For this review, take the finished solid that the model builds, in its own axes (mm). Give positions to 0.01 mm unless a question says otherwise; leave off trailing zeros. Order: outer loops, then holes, each group sorted by start corner. A loop starts at its lowest first (then second) coordinate and runs counter-clockwise, first axis right, second up.
Item 1: For probe 1 along Z at (x, y) = (1, 88.9); probe 2 along Z at (x, y) = (1.9, 17.5); probe 3 along Y at (x, z) = (3.65, -217.5), list the stretches that pass through material, from the lowest coordinate up.
Item 2: Consider section B-B (y = 88.9). Give the boundary of the cut face in (x, z).
Item 3: Consider section A-A (x = 1.8). Give the number of separate pieces and of enclosed holes in the cut face, plus the area to 3 significant figures.
Item 4: Consider section D-D (y = 50.5). Give the boundary of the cut face in (x, z).
Item 5: For P1, Ø1.5, axis at x = 1, z = -73.5, coming from the -Y side; P2, Ø1.2, axis at x = 2.5, y = -133.5, coming from the -Z side; P3, Ø2, axis at x = 1.5, z = -117, coming from the -Y side, all flat-tipped, find the tip position at first contact; note any pin that passes through.
Item 6: Consider section C-C (z = -44.45). Give the boundary of the cut face in (x, y), plus the area to 3 significant figures.
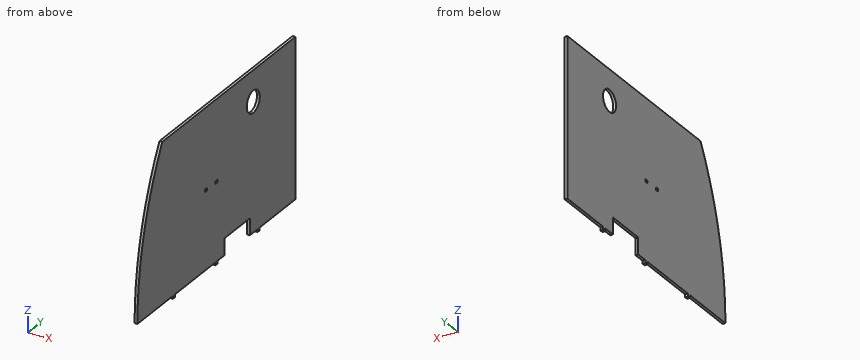
```python
from build123d import *

# Parameters (mm, degrees)
F0_R     = 15.6845
F1_DEPTH = 4.0894
F2_W     = 5.08
F2_H     = 4.0894
F3_DEPTH = 25.4


with BuildPart() as f1:
    # F0 (on Right) → F1 (new body)
    with BuildSketch(Plane.YZ):
        with BuildLine():
            Line((104.3824, -228.6), (190.5, -228.6))
            Line((190.5, -228.6), (190.5, 0))
            Line((190.5, 0), (-130.401722, 0))
            ThreePointArc((-130.401722, 0), (-175.224427, -110.416072), (-190.5, -228.6))
            Line((-190.5, -228.6), (-104.821593, -228.6))
            Line((-104.821593, -228.6), (-99.995593, -228.6))
            Line((-99.995593, -228.6), (-2.54, -228.6))
            Line((-2.54, -228.6), (-2.413, -228.6))
            Line((-2.413, -228.6), (2.413, -228.6))
            Line((2.413, -228.6), (2.54, -228.6))
            Line((2.54, -228.6), (19.796586, -228.6))
            Line((19.796586, -228.6), (19.796586, -204.705998))
            Line((19.796586, -204.705998), (80.546886, -204.705998))
            Line((80.546886, -204.705998), (80.546886, -228.6))
            Line((80.546886, -228.6), (99.06, -228.6))
            Line((99.06, -228.6), (99.3082, -228.6))
            Line((99.3082, -228.6), (104.1342, -228.6))
            Line((104.1342, -228.6), (104.3824, -228.6))
        make_face()
        with Locations((88.9, -44.45)):
            Circle(F0_R, mode=Mode.SUBTRACT)
        Polygon((104.1342, -232.6894), (104.1342, -228.6), (99.3082, -228.6), (99.3082, -232.6894), (101.7212, -232.6894), align=None)
        Polygon((-99.995593, -228.6), (-104.821593, -228.6), (-104.821593, -232.6894), (-102.408593, -232.6894), (-99.995593, -232.6894), align=None)
        Polygon((2.413, -228.6), (-2.413, -228.6), (-2.413, -232.6894), (0, -232.6894), (2.413, -232.6894), align=None)
    extrude(amount=F1_DEPTH)

    # F2 (on face) → F3 (cut)
    with BuildSketch(Plane.YZ.offset(4.0894)):
        with Locations((0, -116.3447)):
            Rectangle(F2_W, F2_H)
        with Locations((-25.4, -116.3447)):
            Rectangle(F2_W, F2_H)
    extrude(amount=-F3_DEPTH, mode=Mode.SUBTRACT)


solid = f1.part
```
Resolved:
1. probe 1: z = -228.6 to -60.13, -28.77 to 0
1. probe 2: z = -228.6 to 0
1. probe 3: y = -190.37 to 19.8, 80.55 to 190.5
2. outline: (0, -228.6) - (4.09, -228.6) - (4.09, -60.13) - (0, -60.13) - close; (0, -28.77) - (4.09, -28.77) - (4.09, 0) - (0, 0) - close
3. separate pieces: 1
3. enclosed holes: 3
3. area: 80,400 mm2
4. outline: (0, -204.71) - (4.09, -204.71) - (4.09, 0) - (0, 0) - close
5. P1: stops at y = -164.12
5. P2: stops at z = -228.6
5. P3: stops at y = -177.15
6. outline: (0, -152.47) - (4.09, -152.47) - (4.09, 73.22) - (0, 73.22) - close; (0, 104.58) - (4.09, 104.58) - (4.09, 190.5) - (0, 190.5) - close
6. area: 1,270 mm2
